Part print with two shaded views. Sizes in mm from the minimum x, y, z corner. Coordinates: 2 decimals unless noted, no trailing zeros. Loops run counter-clockwise (first coordinate to the right, second up) from the corner with the lowest first, then second, coordinate; pieces in that order, holes last. Notation, with made-up numbers: (-1.75, 89.5) - (51.25, 89.5) arc R13 cw to (51.25, 109.5) - close; hole circle Ø6 at (79, 78.25). An arc over 180 degrees is marked (long way). Write each question's results on one line, items separated by ' | '. Start each with the question number.
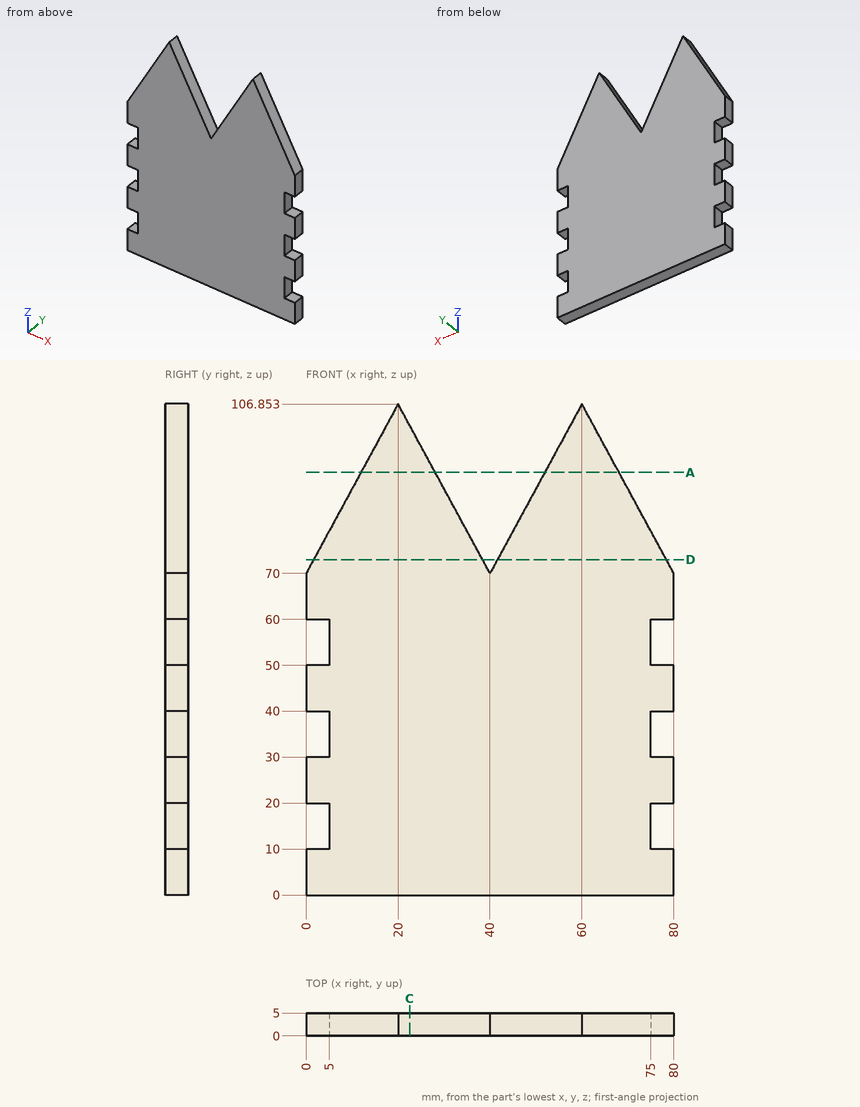
Q1. Cut at A-A (z = 92). List the corners of the cut face in (x, y), and give its area (3 significant figures).
Q2. Drill centre lines: L1, parallel to Z at x = 76.5, y = 0.6; L2, parallel to X at y = 0.4, z = 83 (1 decimal); L3, parallel to X at y = 0.4, z = 53.5. Where is each one in solid material? Low to high. Write a range as from..to.
Q3. Cut at D-D (z = 73). List the corners of the cut face in (x, y).
Q4. Pin check, flat tips, straight feed: pin 1 (3 mm diameter, centred on y = 2.5, z = 72, fed in from -X); pin 2 (3 mm diameter, centred on x = 16.5, y = 0.5, fed in from +Z); pin 3 (1.5 mm diameter, centred on y = 3, z = 36.5, fed in from -X). Stop position of each tip, or through.
Q5. Cut at C-C (x = 22.5). List the corners of the cut face in (y, z), and give its area (3 significant figures).
Check result:
1) outline: (11.94, 0) - (28.06, 0) - (28.06, 5) - (11.94, 5) - close; (51.94, 0) - (68.06, 0) - (68.06, 5) - (51.94, 5) - close | area: 161 mm²
2) L1: 0..10, 20..30, 40..50, 60..76.45 | L2: 7.1..32.9, 47.1..72.9 | L3: 5..75
3) outline: (1.63, 0) - (38.37, 0) - (38.37, 5) - (1.63, 5) - close; (41.63, 0) - (78.37, 0) - (78.37, 5) - (41.63, 5) - close
4) pin 1: x = 0.27 | pin 2: z = 103.17 | pin 3: x = 5
5) outline: (0, 0) - (5, 0) - (5, 102.25) - (0, 102.25) - close | area: 511 mm²
